Could you check a few things on this model? Use its own coordinates, in mm. Face numbers are marked on the shaded views. Coordinates: 2 decimals unless noted, no trailing zeros. Answer as CSV lines item,"result". Start each with the question number.
Item 1: We'd pull the mould along Y, two halves only. Please class the marked faces 1 and 2: +Y half, -Y half, draft (parallel to the pull), parting line (faces both ways), or undercut.
Item 2: If I drill on line 1 along X through (y, z) = (21, 24.5); line 2 along X through (y, z) = (24, 23.75); line 3 along Y through (x, z) = (-17, 18.75), over which ranges is the centre line in solid material (lowest first)? Write a range as [from, to].
Item 3: I'm going to push flat-ended pins straight in: P1, Ø8, axis at y = 2, z = 16.5, coming from the +X side; P2, Ø3, axis at y = 5.5, z = 17, coming from the -X side; P3, Ø2, axis at y = 22, z = 15.5, coming from the -X side; P4, Ø4, axis at x = -10, y = 0, coming from the -Z side. Where does each tip first touch, or does it pass through?
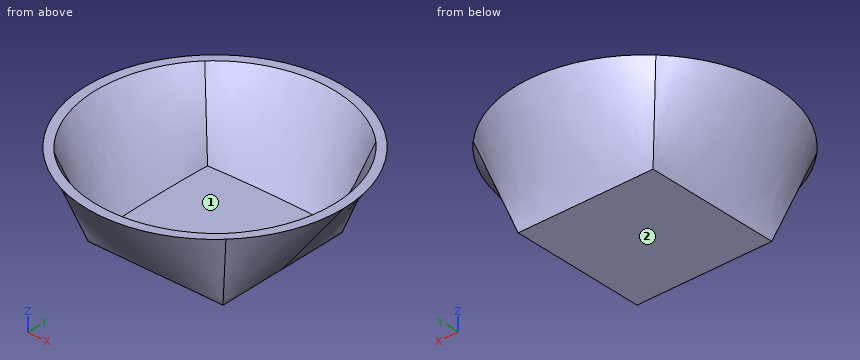
```python
from build123d import *

# Parameters (mm, degrees)
F2_R = 43.0981164558
F1_W = 45
F1_H = 45
F4_T = 2.5


# Not quite as in the source:
# - a shell that OpenCascade refuses in one call is made with other operations: the cavity is built on its own and cut out


with BuildPart() as f3:
    # F2 (on offset) → F3 section 0
    with BuildSketch(Plane.XY.offset(26.7)):
        Circle(F2_R)
    # F1 (on Top) → F3 section 1
    with BuildSketch(Plane.XY):
        Rectangle(F1_W, F1_H)
    loft()

    # F4: shell of thickness 2.5, made by hand


with BuildPart() as f4_core1:
    # F4_t2: copy of F3
    add(f3.part)

    # the walls: a layer under each face that stays
    f4_faces = [f4_core1.faces().sort_by_distance(p)[0] for p in [
        (31.1587338374, 13.8714675651, 13.35),
        (0, 32.7990582263, 13.35),
        (-32.7990582263, 0, 13.35),
        (0, -32.7990582263, 13.35),
        (31.1587338374, -13.8714675651, 13.35),
        (0, 0, 0),
    ]]
    thicken(f4_faces, amount=-F4_T, mode=Mode.SUBTRACT)


with BuildPart() as f3_1:
    add(f3.part)

    # what is left inside the walls is the cavity
    f4_cavity = [f4_core1.part.solids().sort_by_distance(p)[0] for p in [
        (0, -13.313542, 26.675),
    ]]
    add(f4_cavity, mode=Mode.SUBTRACT)


solid = f3_1.part
```
Ans:
1,face 1,"undercut"
1,face 2,"draft"
2,line 1,"x = [-36.11, -32.79], [32.79, 36.11]"
2,line 2,"x = [-33.84, -30.45], [30.45, 33.84]"
2,line 3,"y = [-33.95, -30.79], [30.79, 33.95]"
3,P1,"stops at x = 38.28"
3,P2,"stops at x = -36.48"
3,P3,"stops at x = -30.55"
3,P4,"stops at z = 0"
